The listing builds one solid part. Answer for the finished solid, in the listing's coordinates (mm). A direction names the side the tool comes from. Coordinates: 2 decimals unless noted, no trailing zeros. Loops run counter-clockwise (first coordinate to the right, second up) from the corner with the lowest first, then second, coordinate; pieces in that order, holes last. Notation, with made-up numbers: M -5,-12.75 L 24,-12.75 A21 ccw 24,16.25 Z; hole C 76.5,27 d4. An arc over 180 degrees is marked long. Answer as CSV lines item,"result". Start each with the question number.
```python
from build123d import *

# Parameters (mm, degrees)
ESQUISSE2_W                     = 35
ESQUISSE2_H                     = 35
BOSS_EXTRU_2_DEPTH              = 10
ESQUISSE3_W                     = 22
ESQUISSE3_H                     = 22
ENL_V_DE_MAT_EXTRU_MINCE1_DEPTH = 3
ESQUISSE4_R                     = 5
ENL_V_MAT_EXTRU_1_DEPTH         = 3


with BuildPart() as part:
    # Esquisse2 → Boss.-Extru.2 (new body)
    with BuildSketch(Plane.XY):
        Rectangle(ESQUISSE2_W, ESQUISSE2_H)
    extrude(amount=BOSS_EXTRU_2_DEPTH)

    # Esquisse3 → Enlèv. de mat.-Extru.-Mince1 (cut)
    with BuildSketch(Plane.XY.offset(10)):
        with BuildLine():
            Line((-13, 15), (13, 15))
            ThreePointArc((13, 15), (14.414213562, 14.414213562), (15, 13))
            Line((15, 13), (15, -13))
            ThreePointArc((15, -13), (14.414213562, -14.414213562), (13, -15))
            Line((13, -15), (-13, -15))
            ThreePointArc((-13, -15), (-14.414213562, -14.414213562), (-15, -13))
            Line((-15, -13), (-15, 13))
            ThreePointArc((-15, 13), (-14.414213562, 14.414213562), (-13, 15))
        make_face()
        Rectangle(ESQUISSE3_W, ESQUISSE3_H, mode=Mode.SUBTRACT)
    extrude(amount=-ENL_V_DE_MAT_EXTRU_MINCE1_DEPTH, mode=Mode.SUBTRACT)

    # Esquisse4 → Enlèv. mat.-Extru.1 (cut)
    with BuildSketch(Plane.XY.offset(10)):
        Circle(ESQUISSE4_R)
    extrude(amount=-ENL_V_MAT_EXTRU_1_DEPTH, mode=Mode.SUBTRACT)


solid = part.part
```
Item 1: Section C-C on y = 11.5 is taken. Determine the outline of the cut face in (x, z).
Item 2: For a pull along X with two mould halves and no side action, classify faces 3 (the face through (11, 0, 9)), 4 (the face through (-17.5, 0, 5)), 5 (the face through (-5, 3, 10)) as pulls with the +X half, pulls with the -X half, needs draft (parallel to the pull), parting line crosses it, or undercut.
Item 3: For faces 1 (the face through (0, 15, 9)), 2 (the face through (-16, 0, 10)), determine the directions among +Z, -Z, +X, -X, +Y, -Y from which every point of the face is accessible in a straight line to the end or side of a thin tool.
Item 4: Section A-A on z = 9.25 is taken. Determine the outline of the cut face in (x, y).
Item 5: Consider line 1 (Y direction, x = 0, z = 7.5); line 2 (X direction, y = 5.5, z = 9.5); line 3 (Y direction, x = -2.5, z = 7.25). Determine where each line is inside the solid, lowest interval first.
Item 6: Section B-B on x = 0 is taken. Determine the outline of the cut face in (y, z).
Results are:
1,outline,"M -17.5,0 L 17.5,0 L 17.5,10 L 15,10 L 15,7 L -15,7 L -15,10 L -17.5,10 Z"
2,face 3,"undercut"
2,face 4,"pulls with the -X half"
2,face 5,"needs draft"
3,face 1,"+Z"
3,face 2,"+Z, +X, -X, +Y, -Y"
4,outline,"M -17.5,-17.5 L 17.5,-17.5 L 17.5,17.5 L -17.5,17.5 Z; M -11,-11 L 11,-11 L 11,11 L -11,11 Z; hole M -15,-13 A2 ccw -13,-15 L 13,-15 A2 ccw 15,-13 L 15,13 A2 ccw 13,15 L -13,15 A2 ccw -15,13 Z; hole C 0,0 d10"
5,line 1,"-17.5 to -15, -11 to -5, 5 to 11, 15 to 17.5"
5,line 2,"-17.5 to -15, -11 to 11, 15 to 17.5"
5,line 3,"-17.5 to -15, -11 to -4.33, 4.33 to 11, 15 to 17.5"
6,outline,"M -17.5,0 L 17.5,0 L 17.5,10 L 15,10 L 15,7 L 11,7 L 11,10 L 5,10 L 5,7 L -5,7 L -5,10 L -11,10 L -11,7 L -15,7 L -15,10 L -17.5,10 Z"
